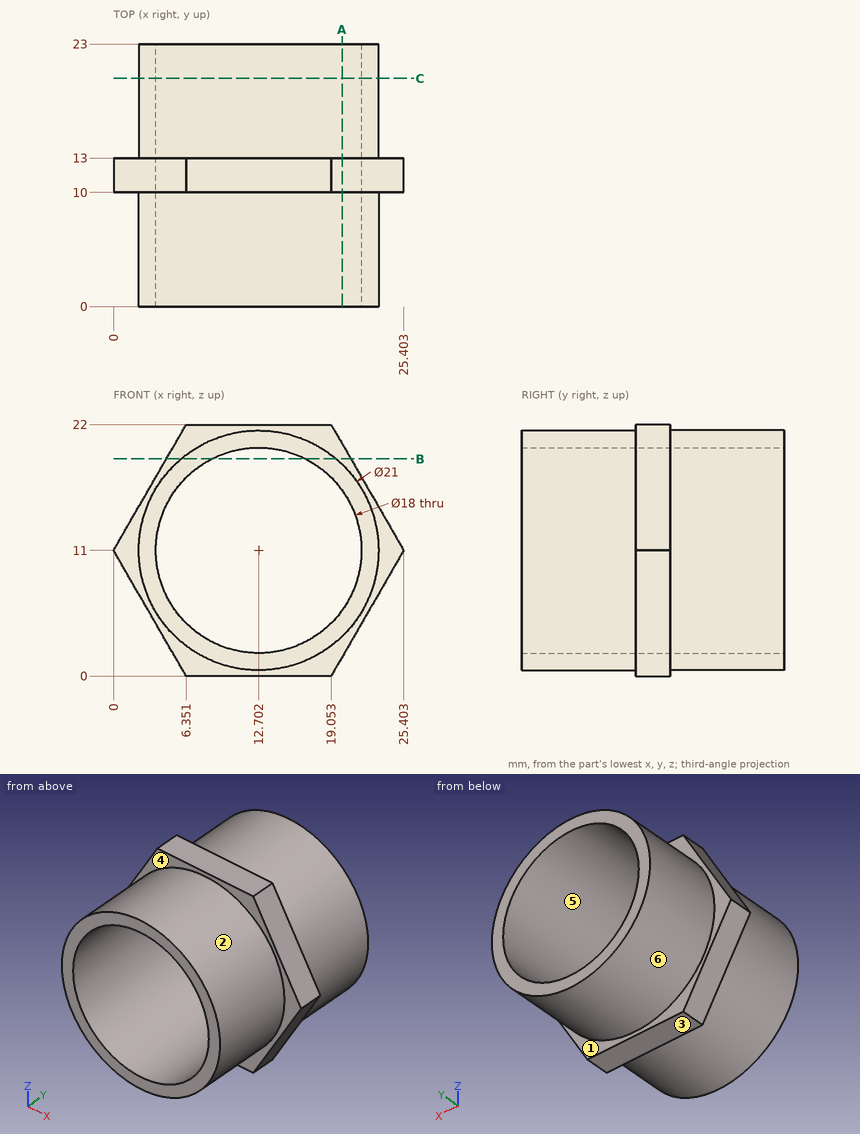
The drawing under review shows one solid part. Ordinate dimensions are in mm from its lowest x, y, z. A direction names the side the tool comes from. Coordinates: 2 decimals unless noted, no trailing zeros. Loops run counter-clockwise (first coordinate to the right, second up) from the corner with the lowest first, then second, coordinate; pieces in that order, holes last.
Item 1: Draft analysis for pull direction Z (two halves, no side actions). For the marked faces 4, 5 and 6, state which applies: pulls with the +Z half, pulls with the -Z half, needs draft (parallel to the pull), parting line crosses it, or undercut.
Completed:
face 4: needs draft
face 5: undercut
face 6: parting line crosses it
Item 2: Clearance check with flat-ended pins moving along their axes: pin 1 (6 mm diameter, centred on x = 3, z = 18, fed in from -Y); pin 2 (3 mm diameter, centred on x = 16.5, y = 3, fed in from -Z) (1 decimal); pin 3 (2 mm diameter, centred on x = 16.5, z = 16, fed in from -Y); pin 4 (4 mm diameter, centred on x = 13.5, y = 3.5, fed in from +Z). State where each tip first meets the part, or that it passes through.
Completed:
pin 1: stops at y = 0
pin 2: stops at z = 0.8
pin 3: passes through
pin 4: stops at z = 21.5
Item 3: Wall thickness on L1, parallel to X at y = 21, z = 10.75 (1 decimal); L2, parallel to Y at x = 18.25, z = 1.75; L3, parallel to Z at x = 11.75, y = 5: over which ranges is each line inside the solid? List them lowest first.
Completed:
L1: x = 2.2 to 3.7, 21.7 to 23.2
L2: y = 10 to 13
L3: z = 0.54 to 2.05, 19.95 to 21.46
Item 4: Add section B-B (z = 19). Write out the cut boundary in (x, y) (1 decimal).
Completed:
outline: (4.6, 10) - (5.9, 10) - (5.9, 0) - (8.6, 0) - (8.6, 23) - (5.9, 23) - (5.9, 13) - (4.6, 13) - close; (16.8, 0) - (19.5, 0) - (19.5, 10) - (20.8, 10) - (20.8, 13) - (19.5, 13) - (19.5, 23) - (16.8, 23) - close
Item 5: For the marked faces 1, 2 and 3, list the 3-axis set-ups (+Z, -Z, +X, -X, +Y, -Y) from which the entire face can be reached by the end or side of a thin tool; tool diameter is ignored.
Completed:
face 1: +Y
face 2: -Y
face 3: -Z, +X, -X, +Y, -Y
Item 6: Add section C-C (y = 20). Write out the cut boundary in (x, z).
Completed:
outline: circle Ø21 at (12.7, 11); hole circle Ø18 at (12.7, 11)
Item 7: Add section A-A (x = 20). Write out the cut boundary in (y, z), and give its area (3 significant figures).
Completed:
outline: (0, 3.45) - (10, 3.45) - (10, 1.64) - (13, 1.64) - (13, 3.45) - (23, 3.45) - (23, 5.73) - (0, 5.73) - close; (0, 16.27) - (23, 16.27) - (23, 18.55) - (13, 18.55) - (13, 20.36) - (10, 20.36) - (10, 18.55) - (0, 18.55) - close
area: 116 mm2
